Could you check a few things on this model? Use its own coordinates, in mm. Face numbers are marked on the shaded views. Coordinates: 2 decimals unless noted, no trailing zeros. Write each loop counter-clockwise with the first axis right and the second up, starting at its lowest first coordinate (ties: lowest second). Pieces come first, ordered by that corner, then holes. Notation, with made-up numbers: M 43,-4 L 58,-4 A34 ccw 58,29 Z; hole C 14.25,32 d4. An arc over 180 degrees is marked long. Write item = value, one per line.
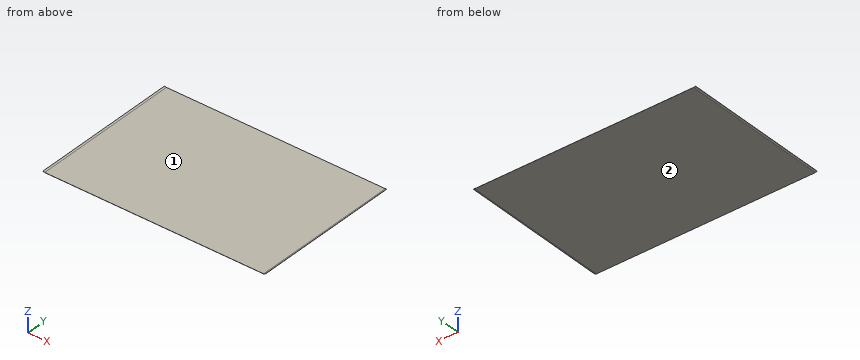
Autodesk Inventor part; units mm, degrees
ref_plane "YZ Plane" through (0, 0, 0) normal (1, 0, 0) x (0, 1, 0)
ref_plane "XZ Plane" through (0, 0, 0) normal (0, 1, 0) x (-1, 0, 0)
ref_plane "XY Plane" through (0, 0, 0) normal (0, 0, 1) x (1, 0, 0)
sketch "Sketch1" plane through (0, 0, 0) normal (0, 0, 1) x (1, 0, 0)
  line L0 (0, 0) -> (1200, 0)
  line L1 (1200, 0) -> (1200, 820)
  line L2 (1200, 820) -> (0, 820)
  line L3 (0, 820) -> (0, 0)
  dimension "d0" = 820
  dimension "d1" = 1200
extrude "Extrusion1" add sketch "Sketch1" along normal blind 0.8
sketch "Sketch4" plane through (0, 0, 0) normal (0, -1, 0) x (1, 0, 0)
  line L0 (1200, 0) -> (0, 0)
  line L1 (0, 0) -> (-9.3969, 3.4202)
  line L2 (0, 0) -> (0, 0.8)
  line L3 (0, 0.8) -> (-9.3969, 4.2202)
  line L4 (-9.3969, 3.4202) -> (-9.3969, 4.2202)
  dimension "d16" = 70
  dimension "d17" = 10
  dimension "d18" = 70
  dimension "d19" = 10
extrude "Extrusion4" add sketch "Sketch4" against normal up to surface (820 mm away)
sketch "Sketch5" plane through (0, 0, 0) normal (0, -1, 0) x (1, 0, 0)
  line L0 (1200, 0) -> (1200, 0.8)
  line L1 (1200, 0) -> (1209.3969, 3.4202)
  line L2 (1200, 0.8) -> (1209.3969, 4.2202)
  line L3 (1209.3969, 3.4202) -> (1209.3969, 4.2202)
  point P0 (0, 0)
  dimension "d22" = 70
  dimension "d23" = 10
  dimension "d24" = 70
  dimension "d25" = 10
extrude "Extrusion5" add sketch "Sketch5" against normal up to surface (820 mm away)
sketch "Sketch7" plane through (0, 0, 0.8) normal (0, 0, 1) x (1, 0, 0)
  circle A0 centre (56.6674, 837.4999) radius 7.5
  line L0 (19.1715, 870) -> (19.1715, -50)
  circle A1 centre (1126.6715, 837.4999) radius 7.5
  line L1 (1159.1715, 870) -> (1159.1715, -50)
  point P0 (0, 0)
  dimension "d30" = 15
  dimension "d31" = 32.5
extrude "Extrusion6" cut sketch "Sketch7" against normal blind 10
ref_plane "Work Plane2" through (0, 410, 0) normal (0, -1, 0) x (1, 0, 0)
mirror "Mirror2" about plane through (0, 410, 0) normal (0, -1, 0) of "Extrusion6"
properties part number "Ke_Bang_Tai"
Item 1: Imagine slicing it at C-C (x = 1051.5). Write out the boundary of the cut face in (y, z).
Numbers:
outline = M 0,0 L 820,0 L 820,0.8 L 0,0.8 Z
Item 2: Imagine slicing it at B-B (z = 2.4). Write out the boundary of the cut face in (x, y).
Numbers:
outline = M -6.59,0 L -4.4,0 L -4.4,820 L -6.59,820 Z; M 1204.4,0 L 1206.59,0 L 1206.59,820 L 1204.4,820 Z
Item 3: If we mould it in two halves opening along X, with no side actions, what happens to the marked faces 1 and 2? For each: pulls with the +X half, pulls with the -X half, needs draft (parallel to the pull), parting line crosses it, or undercut.
Numbers:
face_1 = undercut
face_2 = needs draft
Item 4: If I drill on line 1 along Z through (x, y) = (646, 51), over which ranges is the centre line in solid material (lowest first)?
Numbers:
line_1 = 0 to 0.8
Item 5: Imagine slicing it at A-A (y = 680.5). Write out the boundary of the cut face in (x, z).
Numbers:
outline = M -9.4,3.42 L 0,0 L 1200,0 L 1209.4,3.42 L 1209.4,4.22 L 1200,0.8 L 0,0.8 L -9.4,4.22 Z
